Verification items for the finished model (mm, model axes). Coordinates: 2 decimals unless noted, no trailing zeros. Order: outer loops, then holes, each group sorted by start corner. A loop starts at its lowest first (then second) coordinate and runs counter-clockwise, first axis right, second up. Notation, with made-up numbers: M 44.5,-13 L 55.5,-13 A22 ccw 55.5,15 Z; hole C 48.25,88 d2. An arc over 180 degrees is marked long. Answer as a JSON object with one key per item and string values. Group by question number.
(1) Cross-section at D-D (z = 96.5). Enter the section's corners in (x, y).
(2) Cross-section at B-B (x = 0). Enter the section's corners in (y, z).
(3) Material ranges on line 1 (Z direction, x = -46, y = 115.5); line 2 (Z direction, x = -73, y = 10.5); line 3 (X direction, y = 114.5, z = 16), recorded low to high.
(4) Gauge pin test, flat ends, axial feed: pin 1 Ø6 at (x, z) = (72.5, 51.5) entering from +Y; pin 2 Ø6 at (x, z) = (47.5, -103) entering from +Y; pin 3 Ø12 at (x, y) = (77, 29.5) entering from -Z. Record the tip position at first contact, or that the pin passes through.
(5) Cross-section at A-A (z = 0). Enter the section's corners in (x, y), plus the area to 3 significant figures.
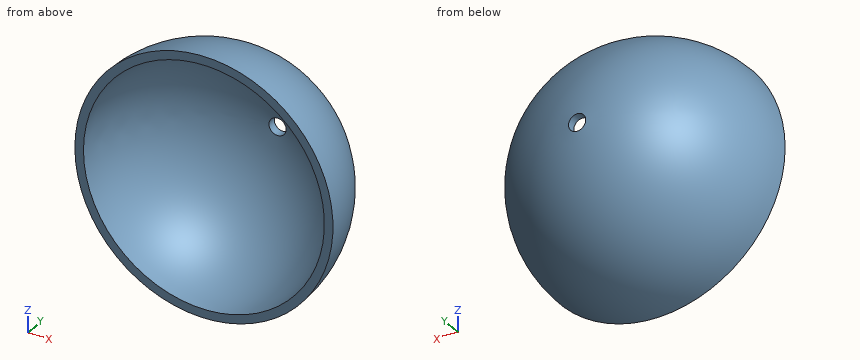
from build123d import *

# Parameters (mm, degrees)
SHELL1_T                = -10
SKETCH2_R               = 10
CUT_EXTRUDE3_DEPTH      = 260.807621135
CUT_EXTRUDE3_DEPTH_BACK = 260.807621135


with BuildPart() as part:
    # Sketch1 → Revolve1 (revolve)
    with BuildSketch(Plane.XY):
        with BuildLine():
            Line((0, 0), (0, 150))
            ThreePointArc((0, 150), (-106.066017178, 106.066017178), (-150, 0))
            Line((-150, 0), (0, 0))
        make_face()
    revolve(axis=Axis((0, 0, 0), (0, 1, 0)))

    # Shell1
    shell1_openings = [part.faces().sort_by_distance(p)[0] for p in [
        (0, 0, 0),
    ]]
    offset(amount=SHELL1_T, openings=shell1_openings, kind=Kind.INTERSECTION)

    # Sketch2 → Cut-Extrude3 (cut, two sides)
    with BuildSketch(Plane(origin=(0, 0, 0), x_dir=(1, 0, 0), z_dir=(0, 1, 0))) as cut_extrude3_sk:
        with Locations(Location((0, 0, 0), (0, 0, 270))):
            Circle(SKETCH2_R)
    extrude(amount=CUT_EXTRUDE3_DEPTH, mode=Mode.SUBTRACT)
    extrude(cut_extrude3_sk.sketch, amount=-CUT_EXTRUDE3_DEPTH_BACK, mode=Mode.SUBTRACT)


solid = part.part
Taken from the geometry:
{
 "1": {"outline": "M -114.84,0 L -101.43,0 A101.43 cw 101.43,0 L 114.84,0 A114.84 ccw Z"},
 "2": {"outline": "M 0,-150 A150 ccw 149.67,-10 L 139.64,-10 A140 cw 0,-140 Z; M 0,140 A140 cw 139.64,10 L 149.67,10 A150 ccw 0,150 Z"},
 "3": {"line 1": "z = -83.93 to -64.37, 64.37 to 83.93", "line 2": "z = -130.62 to -119, 119 to 130.62", "line 3": "x = -95.57 to -78.95, 78.95 to 95.57"},
 "4": {"pin 1": "stops at y = 122.95", "pin 2": "stops at y = 101.52", "pin 3": "stops at z = -129.05"},
 "5": {"outline": "M -150,0 L -140,0 A140 cw -10,139.64 L -10,149.67 A150 ccw Z; M 10,139.64 A140 cw 140,0 L 150,0 A150 ccw 10,149.67 Z", "area": "4,360 mm²"}
}
